```python
from build123d import *

# Parameters (mm, degrees)
SKETCH1_R           = 11
BOSS_EXTRUDE1_DEPTH = 3.5
SKETCH2_R           = 4.05
CUT_EXTRUDE3_DEPTH  = 3
CIRPATTERN1_COUNT   = 8


with BuildPart() as part:
    # Sketch1 → Boss-Extrude1 (new body, symmetric)
    with BuildSketch(Plane.XY):
        Polygon((6.213203436, 15), (-6.213203436, 15), (-15, 6.213203436), (-15, -6.213203436), (-6.213203436, -15), (6.213203436, -15), (15, -6.213203436), (15, 6.213203436), align=None)
        Circle(SKETCH1_R, mode=Mode.SUBTRACT)
    extrude(amount=BOSS_EXTRUDE1_DEPTH, both=True)

    # Sketch2 → Cut-Extrude3 (cut)
    with BuildSketch(Plane(origin=(0, -15, 0), x_dir=(-1, 0, 0), z_dir=(0, -1, 0))):
        Circle(SKETCH2_R)
    cut_extrude3 = extrude(amount=-CUT_EXTRUDE3_DEPTH, mode=Mode.SUBTRACT)

    # CirPattern1: Cut-Extrude3 ×8 about axis
    cirpattern1_axis = Axis((0, 0, 0), (0, 0, 1))
    for i in range(1, CIRPATTERN1_COUNT):
        add(cut_extrude3.rotate(cirpattern1_axis, i * 360 / CIRPATTERN1_COUNT), mode=Mode.SUBTRACT)


solid = part.part
```
Could you check a few things on this model? Use its own coordinates, in mm. A direction names the side the tool comes from. Coordinates: 2 decimals unless noted, no trailing zeros. Write each loop counter-clockwise with the first axis right and the second up, starting at its lowest first coordinate (ties: lowest second). Pieces come first, ordered by that corner, then holes. Notation, with made-up numbers: (52.25, 68.25) -> (75.25, 68.25) arc R24 cw to (75.25, 93.25) -> close; hole circle Ø6 at (-14.5, 66). An arc over 180 degrees is marked (long way). Return JSON: item names as keys, results as strings.
(1) Imagine slicing it at C-C, the plane x = 8.75. Count the separate pieces of the cut face and the enclosed holes in it, then the cut area to 3 significant figures.
Numbers:
{"separate pieces": "6", "enclosed holes": "0", "area": "22.4 mm2"}
(2) Which directions (+Z, -Z, +X, -X, +Y, -Y) give clear straight access to the entire face, cutting with the end or side of a thin tool? Please do faces 5 (the flat face through (15, 5, 0)), 6 (the cylindrical face through (4.05, 13.52, 0.06)), 7 (the cylindrical face through (-13.52, 4.05, 0.06)), 8 (the flat face through (-8.445, -8.525, -0.049)), 9 (the flat face through (12, 0, 0)).
Numbers:
{"face 5": "+Z, -Z, +X, +Y, -Y", "face 6": "+Y", "face 7": "-X", "face 8": "none", "face 9": "+X"}
(3) Imagine slicing it at A-A, the plane x = 0. Please give me the cut outline in (y, z), then the cut area to 3 significant figures.
Numbers:
{"outline": "(-12, -3.5) -> (-11, -3.5) -> (-11, 3.5) -> (-12, 3.5) -> close; (11, -3.5) -> (12, -3.5) -> (12, 3.5) -> (11, 3.5) -> close", "area": "14.0 mm2"}
(4) I need wall thicknesses on L1, parallel to Y at x = 0, z = 1.25; L2, parallel to Y at x = -7.25, z = 0.75; L3, parallel to Y at x = 4.75, z = -1.25. Which ranges of each line are inside material? Lowest first, please.
Numbers:
{"L1": "y = -12 to -11, 11 to 12", "L2": "y = -13.96 to -12.88, -9.72 to -8.27, 8.27 to 9.72, 12.88 to 13.96", "L3": "y = -15 to -9.92, 9.92 to 15"}
(5) We'd pull the mould along X, two halves only. Please class faces 1 (the cylindrical face through (-12.424, 6.697, -0.059)), 2 (the flat face through (0, -12, 0)), 3 (the flat face through (-5, -15, 0)), 4 (the flat face through (-15, -5, 0)): +X half, -X half, draft (parallel to the pull), parting line (faces both ways), or undercut.
Numbers:
{"face 1": "undercut", "face 2": "undercut", "face 3": "draft", "face 4": "-X half"}
(6) I'm going to push flat-ended pins straight in: pin 1 (4 mm diameter, centred on x = -7, y = 4.5, fed in from +Z); pin 2 (1.5 mm diameter, centred on x = 7.5, z = 2, fed in from -Y); pin 3 (3.5 mm diameter, centred on x = -1, z = 1.5, fed in from -Y); pin 4 (1 mm diameter, centred on y = -1, z = 2, fed in from -X). Where does each tip first touch, or does it pass through?
Numbers:
{"pin 1": "passes through", "pin 2": "stops at y = -14.46", "pin 3": "stops at y = -12", "pin 4": "stops at x = -12"}
